from build123d import *

# Parameters (mm, degrees)
CAMERA_CONE_SKETCH_W      = 200
CAMERA_CONE_SKETCH_H      = 112.5
CAMERA_CONE_EXTRUDE_DEPTH = 100
CAMERA_CONE_EXTRUDE_DRAFT = -15
CAMERA_CONE_SHELL_T       = -3
HINGE_EXTRUDE_DEPTH       = 146.410161514
HINGE_HOLE_SKETCH_R       = 20
HINGE_HOLE_CUT_DEPTH      = 146.410161514


with BuildPart() as part:
    # Camera Cone Sketch → Camera Cone Extrude (with draft: the straight prism first)
    with BuildSketch(Plane.XY):
        Rectangle(CAMERA_CONE_SKETCH_W, CAMERA_CONE_SKETCH_H)
    extrude(amount=-CAMERA_CONE_EXTRUDE_DEPTH)
    # Camera Cone Extrude: the draft: its side faces are tilted about the plane it starts from
    camera_cone_extrude_sides = [part.faces().sort_by_distance(p)[0] for p in [
        (-100, 0, -50),
        (0, -56.25, -50),
        (100, 0, -50),
        (0, 56.25, -50),
    ]]
    draft(camera_cone_extrude_sides, Plane.XY, CAMERA_CONE_EXTRUDE_DRAFT)

    # Camera Cone Shell
    camera_cone_shell_openings = [part.faces().sort_by_distance(p)[0] for p in [
        (0, 0, 0),
    ]]
    offset(amount=CAMERA_CONE_SHELL_T, openings=camera_cone_shell_openings, kind=Kind.INTERSECTION)

    # Hinge Sketch → Hinge Extrude (add)
    with BuildSketch(Plane(origin=(73.205080757, 0, 0), x_dir=(0, 0, -1), z_dir=(1, 0, 0))):
        with BuildLine():
            Line((100, 29.455080757), (144.182621135, 29.455080757))
            ThreePointArc((144.182621135, 29.455080757), (173.637701892, 0), (144.182621135, -29.455080757))
            Line((144.182621135, -29.455080757), (100, -29.455080757))
            Line((100, -29.455080757), (100, 29.455080757))
        make_face()
    extrude(amount=-HINGE_EXTRUDE_DEPTH)

    # Hinge Hole Sketch → Hinge Hole Cut (cut)
    with BuildSketch(Plane(origin=(73.205080757, 0, 0), x_dir=(0, 0, -1), z_dir=(1, 0, 0))):
        with Locations((144.182621135, 0)):
            Circle(HINGE_HOLE_SKETCH_R)
    extrude(amount=-HINGE_HOLE_CUT_DEPTH, mode=Mode.SUBTRACT)


solid = part.part
Build history of the part. All positions in model axes, mm. A direction names the side the tool comes from. Round coordinates to 2 decimals unless told otherwise and drop trailing zeros. Write each loop counter-clockwise with the first axis right and the second up, starting at its lowest first coordinate (ties: lowest second). Pieces come first, ordered by that corner, then holes. Notation, with made-up numbers: M -26.75,24.25 L 18.25,24.25 A11 cw 18.25,40.25 Z; hole C 68,-19.75 d5. An arc over 180 degrees is marked long. Answer in a Markdown table with one row per item.
1. Mould opens along Y. For faces 1 (the face through (-1.4, 43.04, -49.3)), 2 (the face through (-1, 0, -97)), 3 (the face through (-1.4, -43.04, -49.3)) say: +Y half, -Y half, draft (parallel to the pull), parting line (faces both ways), or undercut.
Geometry check:
| item | result |
|---|---|
| face 1 | +Y half |
| face 2 | undercut |
| face 3 | -Y half |
2. Flat gauge pins, fed straight in: P1, Ø6, axis at x = 41, z = -152, coming from the -Y side; P2, Ø10, axis at x = -37.5, z = -56, coming from the -Y side; P3, Ø6, axis at x = 45, y = 26, coming from the -Z side. Where does each tip first touch, or does it go through?
Geometry check:
| item | result |
|---|---|
| P1 | y = -29.06 |
| P2 | y = -42.58 |
| P3 | z = -162.58 |
3. Saw through at C-C (z = -74). List the corners of the cut face in (x, y).
Geometry check:
| item | result |
|---|---|
| outline | M -80.17,-36.42 L 80.17,-36.42 L 80.17,36.42 L -80.17,36.42 Z; hole M -77.07,-33.32 L 77.07,-33.32 L 77.07,33.32 L -77.07,33.32 Z |
4. Which spindle directions (+Z, -Z, +X, -X, +Y, -Y) get a long thin tool onto all of the face, cutting with end or side? Do faces 4 (the face through (73.205, 0, -121)), 5 (the face through (-73.205, 0, -121)), 6 (the face through (1, -29.455, -122)), 7 (the face through (-86.97, -0.74, -37.04)), 8 (the face through (1, 29.455, -122)). Say none if no direction does.
Geometry check:
| item | result |
|---|---|
| face 4 | -Z, +X, +Y, -Y |
| face 5 | -Z, -X, +Y, -Y |
| face 6 | -Z, +X, -X, -Y |
| face 7 | +Z |
| face 8 | -Z, +X, -X, +Y |
5. Saw through at A-A (y = 0). List the corners of the cut face in (x, z).
Geometry check:
| item | result |
|---|---|
| outline | M -100,0 L -73.21,-100 L -73.21,-124.18 L 73.21,-124.18 L 73.21,-100 L 100,0 L 96.89,0 L 70.9,-97 L -70.9,-97 L -96.89,0 Z; M -73.21,-173.64 L 73.21,-173.64 L 73.21,-164.18 L -73.21,-164.18 Z |
6. Probe L1, parallel to Z at x = -56, y = -7; L2, parallel to Y at x = 72.5, z = -157; L3, parallel to Y at x = 62, z = -69. List the from-to ranges inside material, lowest first. Write a range as [from, to].
Geometry check:
| item | result |
|---|---|
| L1 | [-172.79, -162.92], [-125.45, -97] |
| L2 | [-26.52, -15.35], [15.35, 26.52] |
| L3 | [-37.76, -34.66], [34.66, 37.76] |
7. Saw through at B-B (x = 51.5). List the corners of the cut face in (y, z), and give its area (3 significant figures).
Geometry check:
| item | result |
|---|---|
| outline | M -56.25,0 L -29.46,-100 L -29.46,-144.18 A29.46 ccw 29.46,-144.18 L 29.46,-100 L 56.25,0 L 53.14,0 L 27.15,-97 L -27.15,-97 L -53.14,0 Z; hole C 0,-144.18 d40 |
| area | 3,490 mm2 |
8. Saw through at D-D (x = 76). List the corners of the cut face in (y, z).
Geometry check:
| item | result |
|---|---|
| outline | M -56.25,0 L -32.25,-89.57 L 32.25,-89.57 L 56.25,0 L 53.14,0 L 32.25,-77.98 L -32.25,-77.98 L -53.14,0 Z |
